```python
from build123d import *

# Parameters (mm, degrees)
F0_W     = 1270
F0_H     = 609.6
F1_DEPTH = 73.152
F2_T     = -2.667
F3_W     = 152.4
F3_H     = 101.6
F3_W_2   = 44.45
F3_H_2   = 25.4
F4_DEPTH = 73.153


with BuildPart() as f1:
    # F0 (on Top) → F1 (new body)
    with BuildSketch(Plane.XY):
        Rectangle(F0_W, F0_H)
    extrude(amount=F1_DEPTH)

    # F2
    f2_openings = [f1.faces().sort_by_distance(p)[0] for p in [
        (0, 0, 0),
    ]]
    offset(amount=F2_T, openings=f2_openings)

    # F3 (on face) → F4 (cut, through all)
    with BuildSketch(Plane.XY.offset(73.152)):
        with Locations((-457.2, 228.6)):
            Rectangle(F3_W, F3_H)
        Polygon((-434.975, 127), (-381, 177.8), (-533.4, 177.8), (-479.425, 127), align=None)
        with Locations((-457.2, 114.3)):
            Rectangle(F3_W_2, F3_H_2)
        with Locations((-279.4, -152.4)):
            Rectangle(F3_W, F3_H)
        Polygon((-257.175, -254), (-203.2, -203.2), (-355.6, -203.2), (-301.625, -254), align=None)
        with Locations((-279.4, -266.7)):
            Rectangle(F3_W_2, F3_H_2)
        with Locations((279.4, -152.4)):
            Rectangle(F3_W, F3_H)
        Polygon((301.625, -254), (355.6, -203.2), (203.2, -203.2), (257.175, -254), align=None)
        with Locations((279.4, -266.7)):
            Rectangle(F3_W_2, F3_H_2)
        with Locations((457.2, 228.6)):
            Rectangle(F3_W, F3_H)
        Polygon((479.425, 127), (533.4, 177.8), (381, 177.8), (434.975, 127), align=None)
        with Locations((457.2, 114.3)):
            Rectangle(F3_W_2, F3_H_2)
    extrude(amount=-F4_DEPTH, mode=Mode.SUBTRACT)


solid = f1.part
```
Design review of the part built by this model. Coordinates are the model's own, in mm. A direction names the side the tool comes from. Coordinates: 2 decimals unless noted, no trailing zeros. Order: outer loops, then holes, each group sorted by start corner. A loop starts at its lowest first (then second) coordinate and runs counter-clockwise, first axis right, second up. Notation, with made-up numbers: (48.25, -3.5) - (75.25, -3.5) arc R21 cw to (75.25, 10.5) - close; hole circle Ø6 at (39, -25.5). An arc over 180 degrees is marked (long way). Answer in a Markdown table with one row per item.
(1) Consider section C-C on x = 232. State the section outline as (y, z) points (3 decimals).
Checked values:
| item | result |
|---|---|
| outline | (-304.8, 0) - (-302.133, 0) - (-302.133, 70.485) - (-230.306, 70.485) - (-230.306, 73.152) - (-304.8, 73.152) - close; (-101.6, 70.485) - (302.133, 70.485) - (302.133, 0) - (304.8, 0) - (304.8, 73.152) - (-101.6, 73.152) - close |
(2) Consider section D-D on x = -59. State the section outline as (y, z) points (3 decimals), plus the area to 3 significant figures.
Checked values:
| item | result |
|---|---|
| outline | (-304.8, 0) - (-302.133, 0) - (-302.133, 70.485) - (302.133, 70.485) - (302.133, 0) - (304.8, 0) - (304.8, 73.152) - (-304.8, 73.152) - close |
| area | 2,000 mm^2 |
(3) The part is to be moulded in two halves that separate along Y. For faces 1 (the flat face through (635, -4, 36)), 2 (the flat face through (-9, -304.8, 36)), 3 (the flat face through (-9, -302.133, 35)), 4 (the flat face through (-9, 304.8, 36)), say which applies: released by +Y, released by -Y, zero draft, split by the parting line, or undercut.
Checked values:
| item | result |
|---|---|
| face 1 | zero draft |
| face 2 | released by -Y |
| face 3 | undercut |
| face 4 | released by +Y |
(4) Wall thickness on line 1 along Y through (x, z) = (-576.5, 37.5); line 2 along X through (y, z) = (213, 57); line 3 along Z through (x, y) = (-129.5, 69.5) (3 decimals): over which ranges is each line inside the solid? List them lowest first. Write a range as from..to.
Checked values:
| item | result |
|---|---|
| line 1 | -304.8..-302.13, 302.13..304.8 |
| line 2 | -635..-632.33, 632.33..635 |
| line 3 | 70.485..73.152 |
(5) For faces 5 (the flat face through (-9, 302.133, 35)), 6 (the flat face through (229.81, -228.244, 71.837)), 7 (the flat face through (-635, -4, 36)), list the 3-axis set-ups (+Z, -Z, +X, -X, +Y, -Y) from which the entire face can be reached by the end or side of a thin tool; tool diameter is ignored.
Checked values:
| item | result |
|---|---|
| face 5 | -Z |
| face 6 | +Z, -Z |
| face 7 | +Z, -Z, -X, +Y, -Y |
(6) Consider section A-A on y = 204. State the section outline as (x, z) points (3 decimals), plus the area to 3 significant figures.
Checked values:
| item | result |
|---|---|
| outline | (-635, 0) - (-632.333, 0) - (-632.333, 70.485) - (-533.4, 70.485) - (-533.4, 73.152) - (-635, 73.152) - close; (-381, 70.485) - (381, 70.485) - (381, 73.152) - (-381, 73.152) - close; (533.4, 70.485) - (632.333, 70.485) - (632.333, 0) - (635, 0) - (635, 73.152) - (533.4, 73.152) - close |
| area | 2,950 mm^2 |
(7) Clearance check with a flat-ended pin moving along its axis: pin 1 (1 mm diameter, centred on x = -55, y = 189.5, fed in from -Z) (3 decimals). State where the tip first meets the part, or that it passes through.
Checked values:
| item | result |
|---|---|
| pin 1 | z = 70.485 |
(8) Consider section B-B on z = 29.5. State the section outline as (x, y) points.
Checked values:
| item | result |
|---|---|
| outline | (-635, -304.8) - (635, -304.8) - (635, 304.8) - (-635, 304.8) - close; hole (-632.33, -302.13) - (632.33, -302.13) - (632.33, 302.13) - (-632.33, 302.13) - close |
